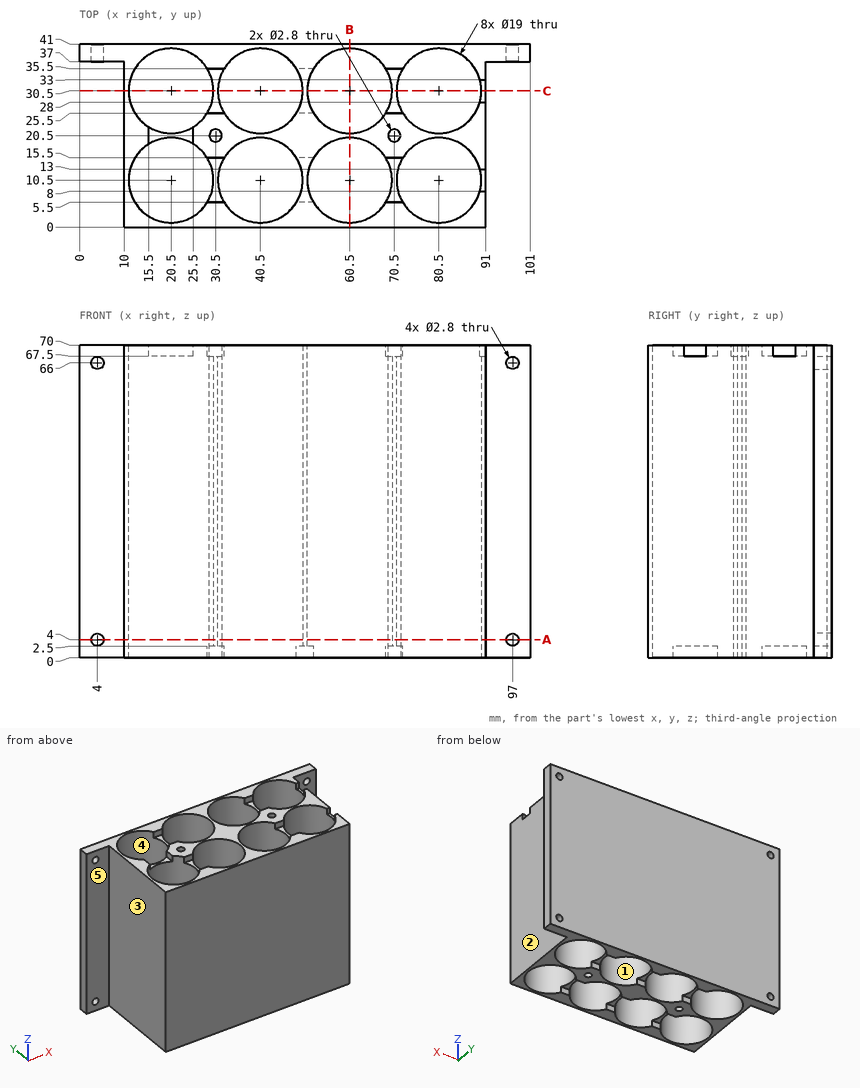
Input: dimensioned drawing with shaded views. Units: mm. Origin: part minimum x, y, z. A direction names the side the tool comes from. Give positions to 0.01 mm unless a question says otherwise; leave off trailing zeros. Write each loop counter-clockwise with the first axis right and the second up, starting at its lowest first coordinate (ties: lowest second). Pieces come first, ordered by that corner, then holes. Notation, with made-up numbers: M -0.5,5 L 35.5,5 A18 cw 35.5,26 Z; hole C -38.5,82.5 d9. An arc over 180 degrees is marked long. Write item = value, one per line. Start each with the question number.
1) Cut plane B-B on x = 60.5. Return the cut outline in (y, z), then the cut area to 3 significant figures.
2) Draft query along X for the marked faces 1, 2 and 3. Return one class per face: +X half, -X half, draft (parallel to the pull), parting line (faces both ways), or undercut.
3) Reachability of the marked faces 4 and 5 from +Z, -Z, +X, -X, +Y, -Y: full face, straight path, thin tool, end or side. Return the list, or none.
4) Cut plane C-C on y = 30.5. Return the cut outline in (x, z), then the cut area to 3 significant figures.
5) Cut plane A-A on z = 4. Count the separate pieces of the cut face and the enclosed holes in it, then the cut area to 3 significant figures.
6) First-contact query: pin 1 Ø1.5 at (y, z) = (14, 46) entering from +X; pin 2 Ø4 at (x, y) = (50, 12) entering from -Z; pin 3 Ø1 at (y, z) = (26.5, 37) entering from -X. Flat tips, straight axial feed; report the tip coordinate or a pass-through.
7) Material intervals for line 1 along X through (y, z) = (10, 48); line 2 along Y through (x, z) = (83.5, 58.5); line 3 along Y through (x, z) = (35.5, 28.5), sorted ascending. Write a range as [from, to].
Solved:
q1.outline = M 0,0 L 1,0 L 1,70 L 0,70 Z; M 20,0 L 21,0 L 21,70 L 20,70 Z; M 40,0 L 41,0 L 41,70 L 40,70 Z
q1.area = 210 mm2
q2.face_1 = undercut
q2.face_2 = +X half
q2.face_3 = -X half
q3.face_4 = +Z, -Z
q3.face_5 = +Z, -Z, -X, -Y
q4.outline = M 10,0 L 11,0 L 11,70 L 10,70 Z; M 30,2.5 L 31,2.5 L 31,67.5 L 30,67.5 Z; M 50,2.5 L 51,2.5 L 51,70 L 50,70 Z; M 70,2.5 L 71,2.5 L 71,67.5 L 70,67.5 Z; M 90,0 L 91,0 L 91,67.5 L 90,67.5 Z
q4.area = 335 mm2
q5.separate_pieces = 3
q5.enclosed_holes = 10
q5.area = 1,100 mm2
q6.pin_1 = 91
q6.pin_2 = 2.5
q6.pin_3 = 10
q7.line_1 = [10, 11.01], [29.99, 31.01], [49.99, 51.01], [69.99, 71.01], [89.99, 91]
q7.line_2 = [0, 1.49], [19.51, 21.49], [39.51, 41]
q7.line_3 = [0, 2.42], [18.58, 22.42], [38.58, 41]
